```python
from build123d import *

# Parameters (mm, degrees)
SKETCH1_W           = 12.7
SKETCH1_H           = 5
BOSS_EXTRUDE1_DEPTH = 2.54
SKETCH2_W           = 0.7
SKETCH2_H           = 0.7
BOSS_EXTRUDE2_DEPTH = 6.7
CHAMFER1_SIZE       = 0.5
CHAMFER2_SIZE       = 0.1


with BuildPart() as part:
    # Sketch1 → Boss-Extrude1 (new body)
    with BuildSketch(Plane.XY):
        Rectangle(SKETCH1_W, SKETCH1_H)
    extrude(amount=BOSS_EXTRUDE1_DEPTH)

    # Sketch2 → Boss-Extrude2 (add)
    with BuildSketch(Plane.XY.offset(2.54)):
        with Locations((-2.54, 1.27)):
            Rectangle(SKETCH2_W, SKETCH2_H)
        with Locations((-5.08, 1.27)):
            Rectangle(SKETCH2_W, SKETCH2_H)
        with Locations((0, 1.27)):
            Rectangle(SKETCH2_W, SKETCH2_H)
        with Locations((2.54, 1.27)):
            Rectangle(SKETCH2_W, SKETCH2_H)
        with Locations((5.08, 1.27)):
            Rectangle(SKETCH2_W, SKETCH2_H)
        with Locations((-2.54, -1.27)):
            Rectangle(SKETCH2_W, SKETCH2_H)
        with Locations((0, -1.27)):
            Rectangle(SKETCH2_W, SKETCH2_H)
        with Locations((2.54, -1.27)):
            Rectangle(SKETCH2_W, SKETCH2_H)
        with Locations((5.08, -1.27)):
            Rectangle(SKETCH2_W, SKETCH2_H)
        with Locations((-5.08, -1.27)):
            Rectangle(SKETCH2_W, SKETCH2_H)
    extrude(amount=BOSS_EXTRUDE2_DEPTH)

    # Chamfer1
    chamfer1_edges = [part.edges().sort_by_distance(p)[0] for p in [
        (6.35, -2.5, 1.27),
        (-6.35, -2.5, 1.27),
        (-6.35, 2.5, 1.27),
        (6.35, 2.5, 1.27),
    ]]
    chamfer(chamfer1_edges, length=CHAMFER1_SIZE)

    # Chamfer2
    chamfer2_edges = [part.edges().sort_by_distance(p)[0] for p in [
        (4.73, -1.27, 9.24),
        (5.08, -1.62, 9.24),
        (5.43, -1.27, 9.24),
        (5.08, -0.92, 9.24),
        (-5.08, -1.62, 9.24),
        (-4.73, -1.27, 9.24),
        (-5.08, -0.92, 9.24),
        (-5.43, -1.27, 9.24),
        (-5.43, 1.27, 9.24),
        (-5.08, 0.92, 9.24),
        (-4.73, 1.27, 9.24),
        (-5.08, 1.62, 9.24),
        (-2.89, 1.27, 9.24),
        (-2.54, 0.92, 9.24),
        (-2.19, 1.27, 9.24),
        (-2.54, 1.62, 9.24),
        (-0.35, 1.27, 9.24),
        (0, 0.92, 9.24),
        (0.35, 1.27, 9.24),
        (0, 1.62, 9.24),
        (2.19, 1.27, 9.24),
        (2.54, 0.92, 9.24),
        (2.89, 1.27, 9.24),
        (2.54, 1.62, 9.24),
        (4.73, 1.27, 9.24),
        (5.08, 0.92, 9.24),
        (5.43, 1.27, 9.24),
        (5.08, 1.62, 9.24),
        (-2.89, -1.27, 9.24),
        (-2.54, -1.62, 9.24),
        (-2.19, -1.27, 9.24),
        (-2.54, -0.92, 9.24),
        (-0.35, -1.27, 9.24),
        (0, -1.62, 9.24),
        (0.35, -1.27, 9.24),
        (0, -0.92, 9.24),
        (2.19, -1.27, 9.24),
        (2.54, -1.62, 9.24),
        (2.89, -1.27, 9.24),
        (2.54, -0.92, 9.24),
    ]]
    chamfer(chamfer2_edges, length=CHAMFER2_SIZE)


solid = part.part
```
Part model, mm, in its own coordinate system. Give positions to 0.01 mm unless a question says otherwise; leave off trailing zeros. Write each loop counter-clockwise with the first axis right and the second up, starting at its lowest first coordinate (ties: lowest second). Pieces come first, ordered by that corner, then holes. Notation, with made-up numbers: (82, -19.75) -> (89, -19.75) arc R15 cw to (89, -13.75) -> close; hole circle Ø10 at (-33.75, -33.75). An arc over 180 degrees is marked (long way). Put each result on its own line as item: value. Start each with the question number.
Item 1: Pin check, flat tips, straight feed: pin 1 Ø1.5 at (y, z) = (-1.5, 5.5) entering from +X; pin 2 Ø0.6 at (x, z) = (-5, 6.5) entering from +Y; pin 3 Ø0.6 at (y, z) = (1, 6.5) entering from -X. Stop position of each tip, or through.
Item 2: Pull direction X, two halves, no side cores. Call faces 1 (the face through (6.35, 0, 1)), 2 (the face through (0, 0, 2.54)), 3 (the face through (-6.35, 0, 1)), 4 (the face through (0, 0, 0)): pulls with the +X half, pulls with the -X half, needs draft (parallel to the pull), parting line crosses it, or undercut.
Item 3: Wall check: L1, parallel to X at y = 1.1, z = 3.25; L2, parallel to Y at x = -0.25, z = 7.75; L3, parallel to Z at x = -3.75, y = -1.3. Give the ranges that are in metal, low to high. Write a range as [from, to].
Item 4: Cut at D-D (y = 0.15). List the corners of the cut face in (x, z).
Item 5: Cut at B-B (z = 4). State how many separate pieces and enclosed holes the cut face has, then the cut area to 3 significant figures.
Item 6: Cut at C-C (x = -4.25). List the corners of the cut face in (y, z), then the cut area to 3 significant figures.
Answer list:
1. pin 1: stops at x = 5.43
1. pin 2: stops at y = 1.62
1. pin 3: stops at x = -5.43
2. face 1: pulls with the +X half
2. face 2: undercut
2. face 3: pulls with the -X half
2. face 4: needs draft
3. L1: x = [-5.43, -4.73], [-2.89, -2.19], [-0.35, 0.35], [2.19, 2.89], [4.73, 5.43]
3. L2: y = [-1.62, -0.92], [0.92, 1.62]
3. L3: z = [0, 2.54]
4. outline: (-6.35, 0) -> (6.35, 0) -> (6.35, 2.54) -> (-6.35, 2.54) -> close
5. separate pieces: 10
5. enclosed holes: 0
5. area: 4.90 mm2
6. outline: (-2.5, 0) -> (2.5, 0) -> (2.5, 2.54) -> (-2.5, 2.54) -> close
6. area: 12.7 mm2
